Read the model definition and answer for the solid it produces. Units are mm, in the model's axes. Give positions to 0.01 mm unless a question says otherwise; leave off trailing zeros. Write each loop counter-clockwise with the first axis right and the second up, starting at its lowest first coordinate (ties: lowest second). Pieces come first, ordered by that corner, then holes. Notation, with made-up numbers: (35, 18) -> (54, 18) arc R17 cw to (54, 30) -> close; hole circle Ø4 at (82.5, 85.5). An arc over 180 degrees is marked (long way). Answer as CSV lines item,"result". Start each with the question number.
1. The part is cut by section A-A, the plane y = 2.5. Determine the outline of the cut face in (x, z).
2. The part is cut by section C-C, the plane z = -8.5. Determine the outline of the cut face in (x, y).
3. The part is cut by section B-B, the plane x = 28.5. Determine the outline of the cut face in (y, z), and give its area (3 significant figures).
4. Given pin 1 (5.5 mm diameter, centred on x = 61.5, z = -3.5, fed in from -Y); pin 2 (2.5 mm diameter, centred on x = 13, z = -2.5, fed in from +Y); pin 3 (1.5 mm diameter, centred on x = 26, y = 2, fed in from -Z), each flat-ended and moving along its own axis, determine where each tip first touches the part or whether it passes through.
5. Find the intervals of material crossed by line 1 (Y direction, x = 100.5, z = -1.5); line 2 (Z direction, x = 9, y = 2.75); line 3 (X direction, y = 0.35, z = -2.5), in increasing order.
from build123d import *

# Parameters (mm, degrees)
SKETCH1_R           = 1
BOSS_EXTRUDE1_DEPTH = 3
FILLET1_R           = 2
BOSS_EXTRUDE2_DEPTH = 0.1
BOSS_EXTRUDE3_DEPTH = 0.1


with BuildPart() as part:
    # Sketch1 → Boss-Extrude1 (new body)
    with BuildSketch(Plane(origin=(0, 0, 0), x_dir=(1, 0, 0), z_dir=(0, 1, 0))):
        Polygon((0, 0), (150, 0), (124.019237886, 45), (124.019237886, 5), (0, 5), align=None)
        with Locations(Location((4, 2.5, 0), (0, 0, 270))):
            Circle(SKETCH1_R, mode=Mode.SUBTRACT)
        with Locations(Location((13, 2.5, 0), (0, 0, 270))):
            Circle(SKETCH1_R, mode=Mode.SUBTRACT)
    extrude(amount=BOSS_EXTRUDE1_DEPTH)

    # Fillet1
    fillet1_edges = [part.edges().sort_by_distance(p)[0] for p in [
        (0, 1.5, -5),
        (0, 1.5, 0),
    ]]
    fillet(fillet1_edges, radius=FILLET1_R)

    # Sketch2 → Boss-Extrude2 (add)
    with BuildSketch(Plane(origin=(0, 3, 0), x_dir=(1, 0, 0), z_dir=(0, 1, 0))):
        Polygon((150, 0), (124.019237886, 45), (124.019237886, 0), align=None)
    extrude(amount=BOSS_EXTRUDE2_DEPTH)

    # Sketch3 → Boss-Extrude3 (add)
    with BuildSketch(Plane.XZ):
        Polygon((124.019237886, -45), (150, 0), (124.019237886, 0), align=None)
    extrude(amount=BOSS_EXTRUDE3_DEPTH)


solid = part.part
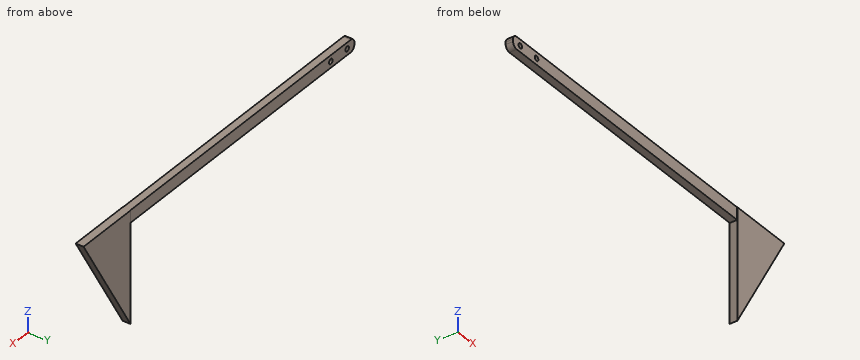
Results found:
1,outline,"(0, -3) arc R2 ccw to (2, -5) -> (124.02, -5) -> (124.02, -45) -> (150, 0) -> (2, 0) arc R2 ccw to (0, -2) -> close; hole circle Ø2 at (4, -2.5); hole circle Ø2 at (13, -2.5)"
2,outline,"(124.02, -0.1) -> (145.09, -0.1) -> (145.09, 3.1) -> (124.02, 3.1) -> close"
3,outline,"(0, -5) -> (3, -5) -> (3, 0) -> (0, 0) -> close"
3,area,"15.0 mm²"
4,pin 1,"stops at y = 0"
4,pin 2,"stops at y = 3"
4,pin 3,"stops at z = -5"
5,line 1,"y = 0 to 3"
5,line 2,"z = -5 to 0"
5,line 3,"x = 0 to 3, 5 to 12, 14 to 148.56"
